```python
from build123d import *

# Parameters (mm, degrees)
BOSS_EXTRUDE1_DEPTH = 17
CUT_EXTRUDE1_REACH  = 77.353
SKETCH2_R           = 3.5
FILLET1_R           = 5


with BuildPart() as part:
    # Sketch1 → Boss-Extrude1 (new body)
    with BuildSketch(Plane.XY):
        with BuildLine():
            Line((-12.5, -11.521718622), (-12.5, -45))
            Line((-12.5, -45), (-30, -45))
            Line((-30, -45), (-30, -50))
            Line((-30, -50), (30, -50))
            Line((30, -50), (30, -45))
            Line((30, -45), (12.5, -45))
            Line((12.5, -45), (12.5, -11.521718622))
            ThreePointArc((12.5, -11.521718622), (0, 17), (-12.5, -11.521718622))
        make_face()
        with BuildLine():
            Line((-3.25, 10.508924778), (-1.758924778, 12))
            Line((-1.758924778, 12), (1.758924778, 12))
            Line((1.758924778, 12), (3.25, 10.508924778))
            ThreePointArc((3.25, 10.508924778), (0, -11), (-3.25, 10.508924778))
        make_face(mode=Mode.SUBTRACT)
    extrude(amount=BOSS_EXTRUDE1_DEPTH)

    # Sketch2 → Cut-Extrude1 (cut, up to next)
    with BuildSketch(Plane.XZ.offset(50), mode=Mode.PRIVATE) as cut_extrude1_sk1:
        with Locations(Location((-22, 8.5, 0), (0, 0, 270))):
            Circle(SKETCH2_R)
    cut_extrude1_tool1 = extrude(cut_extrude1_sk1.sketch, amount=-CUT_EXTRUDE1_REACH, mode=Mode.PRIVATE) & part.part
    # Sketch2 → Cut-Extrude1 (cut, up to next)
    with BuildSketch(Plane.XZ.offset(50), mode=Mode.PRIVATE) as cut_extrude1_sk2:
        with Locations((22, 8.5)):
            Circle(SKETCH2_R)
    cut_extrude1_tool2 = extrude(cut_extrude1_sk2.sketch, amount=-CUT_EXTRUDE1_REACH, mode=Mode.PRIVATE) & part.part
    add(cut_extrude1_tool1.solids().sort_by_distance((-22, -50, 8.5))[0], mode=Mode.SUBTRACT)
    add(cut_extrude1_tool2.solids().sort_by_distance((22, -50, 8.5))[0], mode=Mode.SUBTRACT)

    # Fillet1
    fillet1_edges = [part.edges().sort_by_distance(p)[0] for p in [
        (-12.5, -45, 8.5),
        (-12.5, -11.521718622, 8.5),
        (12.5, -11.521718622, 8.5),
        (12.5, -45, 8.5),
        (-30, -47.5, 17),
        (30, -47.5, 17),
        (30, -47.5, 0),
        (-30, -47.5, 0),
    ]]
    fillet(fillet1_edges, radius=FILLET1_R)


solid = part.part
```
Geometry: final body of the model. Coordinates: model frame, mm. A direction names the side the tool comes from. Round coordinates to 2 decimals unless told otherwise and drop trailing zeros. Order: outer loops, then holes, each group sorted by start corner. A loop starts at its lowest first (then second) coordinate and runs counter-clockwise, first axis right, second up. Notation, with made-up numbers: (55, 41.5) - (112, 41.5) arc R35 cw to (112, 77.5) - close; hole circle Ø8 at (-32.75, 20.25). An arc over 180 degrees is marked (long way). Use CSV: the item, a comma, the result in double quotes. Start each with the question number.
Q1. Section query A-A (z = 8.5). Return loops of the section in (x, y).
Q2. Section query C-C (x = 22). Return loops of the section in (y, z).
Q3. First-contact query: pin 1 (6 mm diameter, centred on x = -25, z = 9, fed in from +Y); pin 2 (3 mm diameter, centred on y = -36, z = 11.5, fed in from -X); pin 3 (8.5 mm diameter, centred on y = -24, z = 5, fed in from +X). Flat tips, straight axial feed; report the tip coordinate or a pass-through.
Q4. Material intervals for line 1 along Z through (x, y) = (22, -48); line 2 along X through (y, z) = (0, 12); line 3 along Y through (x, z) = (20.5, 1.25), sorted ascending. Write a range as from..to.
Q5. Section query B-B (y = 0). Return loops of the section in (x, z).
Q6. Section query D-D (z = 4.25). Return loops of the section in (x, y), and give its area (3 significant figures).
Q7. Mould query, pull axis X, two halves, no side actions, for faces 1 (the face through (28, -47, 1)), 2 (the face through (0, -23, 17)), 3 (the face through (2.494, 11.265, 8.381)). Classes: +X half, -X half, draft (parallel to the pull), parting line (faces both ways), or undercut.
Q8. Access query for faces 4 (the face through (-28, -48, 1)), 5 (the face through (25.2, -45, 10.3)), 6 (the face through (-2.515, 11.244, 8.381)), 7 (the face through (-13.93, -43.5, 8.62)), 8 (the face through (12.77, -11.71, 8.62)). Directions: +Z, -Z, +X, -X, +Y, -Y. A direction counts if a zero-diameter tool reaches every point of the face in a straight line with its end or side. Return the directions, or none.
Result set:
1,outline,"(-30, -50) - (-25.5, -50) - (-25.5, -45) - (-30, -45) - close; (-18.5, -50) - (18.5, -50) - (18.5, -45) - (17.5, -45) arc R5 cw to (12.5, -40) - (12.5, -13.33) arc R5 cw to (13.52, -10.3) arc R17 ccw (long way) to (-13.52, -10.3) arc R5 cw to (-12.5, -13.33) - (-12.5, -40) arc R5 cw to (-17.5, -45) - (-18.5, -45) - close; (25.5, -50) - (30, -50) - (30, -45) - (25.5, -45) - close; hole (-3.25, 10.51) arc R11 ccw (long way) to (3.25, 10.51) - (1.76, 12) - (-1.76, 12) - close"
2,outline,"(-50, 0) - (-45, 0) - (-45, 5) - (-50, 5) - close; (-50, 12) - (-45, 12) - (-45, 17) - (-50, 17) - close"
3,pin 1,"stops at y = -45"
3,pin 2,"stops at x = -12.5"
3,pin 3,"stops at x = 12.5"
4,line 1,"z = 0..5, 12..17"
4,line 2,"x = -17..-11, 11..17"
4,line 3,"y = -50..-45"
5,outline,"(-17, 0) - (-11, 0) - (-11, 17) - (-17, 17) - close; (11, 0) - (17, 0) - (17, 17) - (11, 17) - close"
6,outline,"(-29.94, -50) - (29.94, -50) - (29.94, -45) - (17.5, -45) arc R5 cw to (12.5, -40) - (12.5, -13.33) arc R5 cw to (13.52, -10.3) arc R17 ccw (long way) to (-13.52, -10.3) arc R5 cw to (-12.5, -13.33) - (-12.5, -40) arc R5 cw to (-17.5, -45) - (-29.94, -45) - close; hole (-3.25, 10.51) arc R11 ccw (long way) to (3.25, 10.51) - (1.76, 12) - (-1.76, 12) - close"
6,area,"1,580 mm2"
7,face 1,"+X half"
7,face 2,"draft"
7,face 3,"undercut"
8,face 4,"-Z, -X, +Y, -Y"
8,face 5,"+Z, -Z, +X, +Y"
8,face 6,"+Z, -Z"
8,face 7,"+Z, -Z, -X"
8,face 8,"+Z, -Z, +X"
